Part model, mm, in its own coordinate system. A direction names the side the tool comes from. Give positions to 0.01 mm unless a question says otherwise; leave off trailing zeros. Order: outer loops, then holes, each group sorted by start corner. A loop starts at its lowest first (then second) coordinate and runs counter-clockwise, first axis right, second up. Notation, with made-up numbers: M -8,45.5 L 17,45.5 A26 ccw 17,63.5 Z; hole C 41,10 d11. An arc over 180 degrees is marked long. One line per question, with ' | ' between items.
```python
from build123d import *

# Parameters (mm, degrees)
SKETCH_1_W           = 12.5
SKETCH_1_H           = 48
EXTRUDE_1_DEPTH      = 12.5
EXTRUDE_2_DEPTH      = 2
EXTRUDE_2_DEPTH_BACK = 49.5
SKETCH_2_R           = 0.5


with BuildPart() as part:
    # 草图1 → 凸台-拉伸1 (new body)
    with BuildSketch(Plane.XY):
        Rectangle(SKETCH_1_W, SKETCH_1_H)
    extrude(amount=EXTRUDE_1_DEPTH)

    # 草图2 → 凸台-拉伸2 (add, two sides: drawn at the far end of the back side and taken through both)
    with BuildSketch(Plane(origin=(0, 24, 0), x_dir=(1, 0, 0), z_dir=(0, 1, 0)).offset(-EXTRUDE_2_DEPTH_BACK)):
        with Locations(Location((0, -6.25, 0), (0, 0, 270))):
            Circle(SKETCH_2_R)
    extrude(amount=EXTRUDE_2_DEPTH + EXTRUDE_2_DEPTH_BACK)


solid = part.part
```
1. Slice it at A-A on z = 6.25. Give the cut face in (x, y).
Worked out:
outline: M -6.25,-24 L -0.5,-24 L -0.5,-25.5 L 0.5,-25.5 L 0.5,-24 L 6.25,-24 L 6.25,24 L 0.5,24 L 0.5,26 L -0.5,26 L -0.5,24 L -6.25,24 Z
2. Drop flat-ended pins along their axis: pin 1 (5 mm diameter, centred on x = -4, y = -5, fed in from -Z); pin 2 (3 mm diameter, centred on x = 4, z = 6, fed in from +Y); pin 3 (3 mm diameter, centred on x = -3, z = 6.5, fed in from -Y). Give the stop position or say it passes through.
Worked out:
pin 1: stops at z = 0 | pin 2: stops at y = 24 | pin 3: stops at y = -24
3. Probe L1, parallel to Y at x = 4, z = 10. List the from-to ranges inside material, lowest first. Write a range as from..to.
Worked out:
L1: y = -24..24
4. Slice it at B-B on x = 0. Give the cut face in (y, z), then the cut area to 4 significant figures.
Worked out:
outline: M -25.5,5.75 L -24,5.75 L -24,0 L 24,0 L 24,5.75 L 26,5.75 L 26,6.75 L 24,6.75 L 24,12.5 L -24,12.5 L -24,6.75 L -25.5,6.75 Z | area: 603.5 mm2
5. Tool access for faces 1 (the cylindrical face through (-0.3, -24.76, 5.85)), 2 (the cylindrical face through (-0.3, 24.99, 5.85)), 3 (the flat face through (-6.25, 0, 6)): list every direction of +Z, -Z, +X, -X, +Y, -Y with a clear straight run to the whole face (end or side of a thin tool).
Worked out:
face 1: -Y | face 2: +Y | face 3: +Z, -Z, -X, +Y, -Y
